Check sheet for the modelled part. Datum: model origin and axes. Units: mm. A direction names the side the tool comes from. Give positions to 0.01 mm unless a question says otherwise; leave off trailing zeros. Loops run counter-clockwise (first coordinate to the right, second up) from the corner with the lowest first, then second, coordinate; pieces in that order, holes last. Notation, with made-up numbers: (74, -5.75) - (111, -5.75) arc R38 ccw to (111, 32.25) - close; hole circle Ø6 at (-21, -15). An arc over 180 degrees is marked (long way). Use one line per item in the form item = value.
Autodesk Inventor part; units mm, degrees
ref_plane "YZ Plane" through (0, 0, 0) normal (1, 0, 0) x (0, 1, 0)
ref_plane "XZ Plane" through (0, 0, 0) normal (0, 1, 0) x (-1, 0, 0)
ref_plane "XY Plane" through (0, 0, 0) normal (0, 0, 1) x (1, 0, 0)
sketch "Sketch1" plane through (0, 0, 0) normal (0, 1, 0) x (-1, 0, 0)
  line L0 (21, 5) -> (-21, 5)
  line L1 (-21, 5) -> (-21, -5)
  line L2 (-21, -5) -> (21, -5)
  line L3 (21, -5) -> (21, 5)
  point P0 (0, 0)
  point P1 (21, 0)
  point P2 (0, -5)
  point P3 (17, 0)
  point P4 (0, 0)
  point P5 (-17, 0)
  dimension "d0" = 42
  dimension "d1" = 10
  dimension "d2" = 17
  dimension "d3" = 17
extrude "Extrusion1" add sketch "Sketch1" along normal blind 1.6
sketch "Sketch2" plane through (0, 1.6, 0) normal (0, 1, 0) x (1, 0, 0)
  point P0 (0, 0)
  point P1 (-17, 0)
  point P2 (0, 0)
  point P3 (17, 0)
hole "Hole1" at (-17, 1.6, 0) at (0, 1.6, 0) at (17, 1.6, 0) direction (0, -1, 0) diameter 1 end through all
sketch "Sketch3" plane through (0, 1.6, 0) normal (0, 1, 0) x (1, 0, 0)
  line L0 (-21, -5) -> (21, -5)
  line L1 (-21, -5) -> (21, -5)
  line L2 (-8.5, 0.5052) -> (-8.5, -1.9497) construction
  line L3 (8.5, -1.3927) -> (8.5, 1.0622) construction
  arc A0 (-6, -4) -> (-11, -4) centre (-8.5, -4) ccw
  arc A1 (11, -4) -> (6, -4) centre (8.5, -4) ccw
  line L4 (-11, -4) -> (-11, -5)
  line L5 (-6, -4) -> (-6, -5)
  line L6 (6, -4) -> (6, -5)
  line L7 (11, -4) -> (11, -5)
  point P0 (0, 0)
  dimension "d15" = 17
  dimension "d16" = 8.5
  dimension "d21" = 5
  dimension "d22" = 1
extrude "Extrusion2" cut sketch "Sketch3" against normal blind 1.6
properties part number "Pinhole_insert_1mm_3x"
Item 1: Thickness scan on L1, parallel to X at y = 0.65, z = 0; L2, parallel to X at y = 1.25, z = 4.75; L3, parallel to Z at x = 17, y = 1.25. Record the ranges inside material, lowest first.
Answer block:
L1 = -21 to -17.5, -16.5 to -0.5, 0.5 to 16.5, 17.5 to 21
L2 = -21 to -11, -6 to 6, 11 to 21
L3 = -5 to -0.5, 0.5 to 5
Item 2: Section check D-D on x = 8.5. Record the boundary of the cut face in (y, z).
Answer block:
outline = (0, -5) - (1.6, -5) - (1.6, 1.5) - (0, 1.5) - close
Item 3: Access from +Z, -Z, +X, -X, +Y, -Y to the whole of each face (thin tool, end or side, straight path). Record for faces 4 (the face through (-17.496, 0.789, -0.065)), 5 (the face through (-11, 0.8, 4.5)).
Answer block:
face_4 = +Y, -Y
face_5 = +Z, +Y, -Y
Item 4: Section check A-A on x = 17. Record the boundary of the cut face in (y, z), then the cut area to 3 significant figures.
Answer block:
outline = (0, -5) - (1.6, -5) - (1.6, -0.5) - (0, -0.5) - close; (0, 0.5) - (1.6, 0.5) - (1.6, 5) - (0, 5) - close
area = 14.4 mm2
Item 5: Section check B-B on y = 1.3. Record the boundary of the cut face in (x, z).
Answer block:
outline = (-21, -5) - (21, -5) - (21, 5) - (11, 5) - (11, 4) arc R2.5 cw to (6, 4) - (6, 5) - (-6, 5) - (-6, 4) arc R2.5 cw to (-11, 4) - (-11, 5) - (-21, 5) - close; hole circle Ø1 at (-17, 0); hole circle Ø1 at (0, 0); hole circle Ø1 at (17, 0)
Item 6: Mould release check, pull along X, two halves, no side actions. Record for faces 1 (the face through (8.6, 0.8, 1.5)), 2 (the face through (-21, 1, 0)), 3 (the face through (-16, 1, 5)): released by +X, released by -X, zero draft, split by the parting line, or undercut.
Answer block:
face_1 = undercut
face_2 = released by -X
face_3 = zero draft
Item 7: Section check C-C on z = 2.75. Record the boundary of the cut face in (x, y), then the cut area to 3 significant figures.
Answer block:
outline = (-21, 0) - (-10.67, 0) - (-10.67, 1.6) - (-21, 1.6) - close; (-6.33, 0) - (6.33, 0) - (6.33, 1.6) - (-6.33, 1.6) - close; (10.67, 0) - (21, 0) - (21, 1.6) - (10.67, 1.6) - close
area = 53.3 mm2
